Work out the finished part from the listing and answer in its coordinate system (mm). A direction names the side the tool comes from. Coordinates: 2 decimals unless noted, no trailing zeros. Write each loop counter-clockwise with the first axis right and the second up, starting at its lowest first coordinate (ties: lowest second). Pieces come first, ordered by that corner, then holes. Notation, with made-up numbers: M -16.75,20 L 21.25,20 A21 cw 21.25,40 Z; hole C -38.75,53 d11. An arc over 180 degrees is marked long. Use CSV: the item, a comma, the result in double quotes.
from build123d import *

# Parameters (mm, degrees)
PART2_1_START         = -21.745
PART2_1_OUTLINE_R     = 2.268804718
PART2_1_DEPTH         = 3
PART2_1_START_2       = -18.745
PART2_1_2_OUTLINE_R   = 1.538851722
PART2_1_2_OUTLINE_R_2 = 3.540835997
PART2_1_2_OUTLINE_R_3 = 2.268804718
PART2_1_2_DEPTH       = 5
SKETCH_1_W            = 9.919146705
SKETCH_1_H            = 22.592426062
CUT_EXTRUDE_1_DEPTH   = 1


# Read off the part's stored shape, not the designer's step: 基体零件-part2-1
with BuildPart() as part:
    # 基体零件-part2-1 outline → 基体零件-part2-1 (new body)
    with BuildSketch(Plane.XY.offset(PART2_1_START)):
        with BuildLine():
            ThreePointArc((-0.73742282, -6.986834522), (-1.194921758, -5.497574164), (-2.33759914, -4.438569872))
            ThreePointArc((-2.33759914, -4.438569872), (-5.0165, 0), (-2.33759914, 4.438569872))
            ThreePointArc((-2.33759914, 4.438569872), (-1.194921758, 5.497574164), (-0.73742282, 6.986834522))
            ThreePointArc((-0.73742282, 6.986834522), (-4.313555127, 12.746389448), (-10.998808821, 11.620077647))
            ThreePointArc((-10.998808821, 11.620077647), (-16, 0), (-10.998808821, -11.620077647))
            ThreePointArc((-10.998808821, -11.620077647), (-4.313555127, -12.746389448), (-0.73742282, -6.986834522))
        make_face()
        with Locations((-9.916654285, 0)):
            Circle(PART2_1_OUTLINE_R, mode=Mode.SUBTRACT)
    extrude(amount=PART2_1_DEPTH)

    # part2-1 2 outline → part2-1 2 (add)
    # profile 1 of 3: a face of its own
    with BuildSketch(Plane.XY.offset(PART2_1_START_2)):
        with Locations((-6.816961539, -7.2020183)):
            Circle(PART2_1_2_OUTLINE_R)
    # profile 2 of 3: a face of its own
    with BuildSketch(Plane.XY.offset(PART2_1_START_2)):
        with Locations((-9.916654285, 0)):
            Circle(PART2_1_2_OUTLINE_R_2)
        with Locations((-9.916654285, 0)):
            Circle(PART2_1_2_OUTLINE_R_3, mode=Mode.SUBTRACT)
    # profile 3 of 3: a face of its own
    with BuildSketch(Plane.XY.offset(PART2_1_START_2)):
        with Locations((-6.816961539, 7.2020183)):
            Circle(PART2_1_2_OUTLINE_R)
    extrude(amount=PART2_1_2_DEPTH)

    # 草图1 → 切除-拉伸1 (cut)
    with BuildSketch(Plane.XY.offset(-13.745)):
        with Locations((-9.361869936, 0)):
            Rectangle(SKETCH_1_W, SKETCH_1_H)
    extrude(amount=-CUT_EXTRUDE_1_DEPTH, mode=Mode.SUBTRACT)


solid = part.part
Item 1: The part is cut by section A-A (z = -19.5). Write down the section's boundary in (x, y).
Answer:
outline,"M -11,-11.62 A6.08 ccw -0.74,-6.99 A3 ccw -2.34,-4.44 A5.02 cw -2.34,4.44 A3 ccw -0.74,6.99 A6.08 ccw -11,11.62 A16 ccw Z; hole C -9.92,0 d4.54"
Item 2: The part is cut by section D-D (y = 3.25). Write down the section's boundary in (x, z) (3 decimals), then the cut area to 3 significant figures.
Answer:
outline,"M -15.666,-21.745 L -3.821,-21.745 L -3.821,-18.745 L -8.511,-18.745 L -8.511,-14.745 L -11.322,-14.745 L -11.322,-18.745 L -15.666,-18.745 Z"
area,"46.8 mm2"
Item 3: The part is cut by section C-C (z = -15.75). Write down the section's boundary in (x, y).
Answer:
outline,"C -9.92,0 d7.08; C -6.82,-7.2 d3.08; C -6.82,7.2 d3.08; hole C -9.92,0 d4.54"
Item 4: A tool of negligible diameter and unlimited length cuts with its end or side. For faces 1 (the face through (-9.18, -2.31, -14.745)), 2 (the face through (-1.18, -5.52, -20.27)), 3 (the face through (-6.107, 5.837, -16.773)), from which of +Z, -Z, +X, -X, +Y, -Y can it reach the whole face along a straight path? Write none if from no direction.
Answer:
face 1,"+Z, +X, -X, +Y, -Y"
face 2,"+Z, -Z, +X"
face 3,"+Z"
Item 5: The part is cut by section B-B (y = 0). Write down the section's boundary in (x, z) (1 decimal).
Answer:
outline,"M -16,-21.7 L -12.2,-21.7 L -12.2,-14.7 L -13.5,-14.7 L -13.5,-18.7 L -16,-18.7 Z; M -7.6,-21.7 L -5,-21.7 L -5,-18.7 L -6.4,-18.7 L -6.4,-14.7 L -7.6,-14.7 Z"
Item 6: Given pin 1 (1.5 mm diameter, centred on x = -2.5, z = -17, fed in from -Y); pin 2 (5 mm diameter, centred on x = -12, y = -8, fed in from +Z) (3 decimals), each flat-ended and moving along its own axis, determine where each tip first touches the part or whether it passes through.
Answer:
pin 1,"passes through"
pin 2,"stops at z = -18.745"
Item 7: Consider probe 1 along X at (y, z) = (0, -18.25); probe 2 along X at (y, z) = (0, -19.75); probe 3 along Z at (x, y) = (-7, 5.5) (3 decimals). Determine where each line is inside the solid, lowest interval first.
Answer:
probe 1,"x = -13.46 to -12.19, -7.65 to -6.38"
probe 2,"x = -16 to -12.19, -7.65 to -5.02"
probe 3,"z = -21.745 to -18.745"
Item 8: For a pull along Y with two mould halves and no side action, classify faces 4 (the face through (-16, 0, -20)), 5 (the face through (-11.7, -1.4, -18.3)), 6 (the face through (-7, -7, -14.745)) as released by +Y, released by -Y, zero draft, split by the parting line, or undercut.
Answer:
face 4,"split by the parting line"
face 5,"undercut"
face 6,"zero draft"
